Input: part model. Units: mm. Frame: model coordinates. Face numbers are marked on the shaded views. A direction names the side the tool comes from. Give positions to 0.01 mm unless a question says otherwise; leave off trailing zeros. Order: outer loops, then holes, each group sorted by start corner. A loop starts at its lowest first (then second) coordinate and runs counter-clockwise, first axis right, second up. Notation, with made-up numbers: M 77,75.25 L 130,75.25 A10 ccw 130,82.25 Z; hole C 46,67 d10. An arc over 180 degrees is marked long. Use a Markdown table: item, result.
from build123d import *

# Parameters (mm, degrees)
ESQUISSE1_W             = 35
ESQUISSE1_H             = 27
BOSS_EXTRU_1_DEPTH      = 11
ESQUISSE2_W             = 29
ESQUISSE2_H             = 21
ENL_V_MAT_EXTRU_1_DEPTH = 8
CHANFREIN1_SIZE         = 4
ESQUISSE3_R             = 1
ENL_V_MAT_EXTRU_2_DEPTH = 7
ESQUISSE4_R             = 1
BOSS_EXTRU_2_DEPTH      = 6
CONG_2_R                = 1
CONG_3_R                = 2
CONG_4_R                = 2
ESQUISSE5_W             = 6
ESQUISSE5_H             = 3
ENL_V_MAT_EXTRU_3_DEPTH = 2


with BuildPart() as part:
    # Esquisse1 → Boss.-Extru.1 (new body)
    with BuildSketch(Plane.XY):
        Rectangle(ESQUISSE1_W, ESQUISSE1_H)
    extrude(amount=BOSS_EXTRU_1_DEPTH)

    # Esquisse2 → Enl_v. mat.-Extru.1 (cut)
    with BuildSketch(Plane.XY.offset(11)):
        Rectangle(ESQUISSE2_W, ESQUISSE2_H)
    extrude(amount=-ENL_V_MAT_EXTRU_1_DEPTH, mode=Mode.SUBTRACT)

    # Chanfrein1
    chanfrein1_edges = [part.edges().sort_by_distance(p)[0] for p in [
        (-14.5, -10.5, 7),
        (-14.5, 10.5, 7),
        (14.5, 10.5, 7),
        (14.5, -10.5, 7),
    ]]
    chamfer(chanfrein1_edges, length=CHANFREIN1_SIZE)

    # Esquisse3 → Enl_v. mat.-Extru.2 (cut)
    with BuildSketch(Plane.XY.offset(11)):
        with Locations((-14.5, 10.5)):
            Circle(ESQUISSE3_R)
        with Locations((14.5, 10.5)):
            Circle(ESQUISSE3_R)
        with Locations((14.5, -10.5)):
            Circle(ESQUISSE3_R)
        with Locations((-14.5, -10.5)):
            Circle(ESQUISSE3_R)
    extrude(amount=-ENL_V_MAT_EXTRU_2_DEPTH, mode=Mode.SUBTRACT)

    # Esquisse4 → Boss.-Extru.2 (add)
    with BuildSketch(Plane.XY.offset(3)):
        with Locations((-8.1, 7.5)):
            Circle(ESQUISSE4_R)
        with Locations((8.1, 7.5)):
            Circle(ESQUISSE4_R)
        with Locations((-8.1, -7.5)):
            Circle(ESQUISSE4_R)
        with Locations((8.1, -7.5)):
            Circle(ESQUISSE4_R)
    extrude(amount=BOSS_EXTRU_2_DEPTH)

    # Cong_2
    cong_2_edges = [part.edges().sort_by_distance(p)[0] for p in [
        (-9.1, 7.5, 9),
        (7.1, 7.5, 9),
        (-9.1, -7.5, 9),
        (7.1, -7.5, 9),
    ]]
    fillet(cong_2_edges, radius=CONG_2_R)

    # Cong_3
    cong_3_edges = [part.edges().sort_by_distance(p)[0] for p in [
        (-17.5, 13.5, 5.5),
        (17.5, 13.5, 5.5),
        (17.5, -13.5, 5.5),
        (-17.5, -13.5, 5.5),
    ]]
    fillet(cong_3_edges, radius=CONG_3_R)

    # Cong_4
    cong_4_edges = [part.edges().sort_by_distance(p)[0] for p in [
        (10.5, -10.5, 7),
        (-10.5, -10.5, 7),
        (-14.5, 6.5, 7),
        (-14.5, -6.5, 7),
        (14.5, 6.5, 7),
        (14.5, -6.5, 7),
        (-10.5, 10.5, 7),
        (10.5, 10.5, 7),
    ]]
    fillet(cong_4_edges, radius=CONG_4_R)

    # Esquisse5 → Enl_v. mat.-Extru.3 (cut)
    with BuildSketch(Plane.XY.offset(11)):
        with Locations((0, 12)):
            Rectangle(ESQUISSE5_W, ESQUISSE5_H)
    extrude(amount=-ENL_V_MAT_EXTRU_3_DEPTH, mode=Mode.SUBTRACT)


solid = part.part
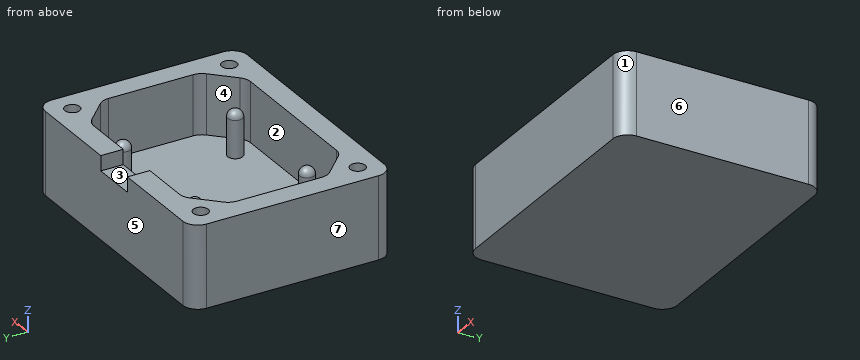
1) First-contact query: pin 1 Ø1.8 at (x, y) = (14.5, 10.5) entering from +Z; pin 2 Ø4 at (x, y) = (5, -4) entering from +Z. Flat tips, straight axial feed; report the tip coordinate or a pass-through.
Response values:
| item | result |
|---|---|
| pin 1 | stops at z = 4 |
| pin 2 | stops at z = 3 |
2) Reachability of the marked faces 1, 2 and 3 from +Z, -Z, +X, -X, +Y, -Y: full face, straight path, thin tool, end or side. Return the list, or none.
Response values:
| item | result |
|---|---|
| face 1 | +Z, -Z, +X, -Y |
| face 2 | +Z |
| face 3 | +Z, +Y |
3) Cut plane C-C on y = 2. Return loops of the section in (x, z).
Response values:
| item | result |
|---|---|
| outline | M -17.5,0 L 17.5,0 L 17.5,11 L 14.5,11 L 14.5,3 L -14.5,3 L -14.5,11 L -17.5,11 Z |
4) Mould query, pull axis X, two halves, no side actions, for the marked faces 4, 5, 6 and 7. Classes: released by +X, released by -X, zero draft, split by the parting line, or undercut.
Response values:
| item | result |
|---|---|
| face 4 | undercut |
| face 5 | zero draft |
| face 6 | released by +X |
| face 7 | released by -X |
5) Cut plane B-B on x = 8.1. Return loops of the section in (y, z).
Response values:
| item | result |
|---|---|
| outline | M -13.5,0 L 13.5,0 L 13.5,11 L 10.5,11 L 10.5,3 L 8.5,3 L 8.5,8 A1 ccw 6.5,8 L 6.5,3 L -6.5,3 L -6.5,8 A1 ccw -8.5,8 L -8.5,3 L -10.5,3 L -10.5,11 L -13.5,11 Z |
6) Material intervals for line 1 (Y direction, x = 4.5, z = 6.75); line 2 (X direction, y = 3, z = 9); line 3 (X direction, y = 8, z = 3.75), sorted ascending. Write a range as from..to.
Response values:
| item | result |
|---|---|
| line 1 | y = -13.5..-10.5, 10.5..13.5 |
| line 2 | x = -17.5..-14.5, 14.5..17.5 |
| line 3 | x = -17.5..-13, -8.97..-7.23, 7.23..8.97, 13..17.5 |
7) Cut plane A-A on z = 4.5. State how many separate pieces and enclosed holes the cut face has, and give its area (3 significant figures).
Response values:
| item | result |
|---|---|
| separate pieces | 5 |
| enclosed holes | 5 |
| area | 365 mm² |
